For this review, take the finished solid that the model builds, in its own axes (mm). A direction names the side the tool comes from. Coordinates: 2 decimals unless noted, no trailing zeros. Loops run counter-clockwise (first coordinate to the right, second up) from the corner with the lowest first, then second, coordinate; pieces in that order, holes last. Notation, with made-up numbers: (-9, 6.5) -> (39, 6.5) arc R37 ccw to (39, 45.5) -> close; hole circle Ø9 at (7.25, -24). An arc over 180 degrees is marked (long way). Answer in a Markdown table with one row per item.
Autodesk Inventor part; units mm, degrees
ref_plane "YZ Plane" through (0, 0, 0) normal (1, 0, 0) x (0, 1, 0)
ref_plane "XZ Plane" through (0, 0, 0) normal (0, 1, 0) x (-1, 0, 0)
ref_plane "XY Plane" through (0, 0, 0) normal (0, 0, 1) x (1, 0, 0)
sketch "Sketch1" plane through (0, 0, 0) normal (0, 1, 0) x (-1, 0, 0)
  line L0 (0, 0) -> (12.7, 0)
  line L1 (12.7, 0) -> (12.7, 38.1)
  line L2 (12.7, 38.1) -> (0, 38.1)
  line L3 (0, 38.1) -> (0, 0)
  circle A0 centre (6.35, 31.75) radius 2.5797
  circle A1 centre (6.35, 6.35) radius 2.5797
  line L4 (0, 0) -> (127, 0)
  line L5 (127, 0) -> (127, 3.175)
  line L6 (127, 3.175) -> (0, 3.175)
  line L7 (0, 3.175) -> (0, 0)
  line L8 (12.7, 38.1) -> (127, 3.175)
  line L9 (0, 3.175) -> (127, 3.175)
  line L10 (127, 3.175) -> (127, 1.5875)
  line L11 (127, 1.5875) -> (0, 1.5875)
  line L12 (0, 1.5875) -> (0, 3.175)
  line L13 (0, 3.175) -> (19.05, 3.175)
  line L14 (19.05, 3.175) -> (19.05, 1.5875)
  line L15 (19.05, 1.5875) -> (0, 1.5875)
  line L16 (0, 1.5875) -> (0, 3.175)
  line L17 (127, 3.175) -> (120.65, 3.175)
  line L18 (120.65, 3.175) -> (120.65, 1.5875)
  line L19 (120.65, 1.5875) -> (127, 1.5875)
  line L20 (127, 1.5875) -> (127, 3.175)
  line L21 (120.65, 3.175) -> (120.65, 5.1153)
  line L22 (127, 0) -> (0, 0)
  line L23 (0, 0) -> (0, -12.7)
  line L24 (0, -12.7) -> (127, -12.7)
  line L25 (127, -12.7) -> (127, 0)
  line L26 (120.65, 1.5875) -> (120.65, 0)
  line L27 (19.05, 1.5875) -> (19.05, 0)
  point P0 (0, 3.175)
  point P1 (0, 1.5875)
  point P2 (120.65, 1.5875)
  point P3 (120.65, 3.175)
  point P4 (19.05, 3.175)
  point P5 (19.05, 1.5875)
  point P6 (120.65, 3.175)
  point P7 (12.7, 1.5875)
  point P8 (12.7, 3.175)
  dimension "d0" = 12.7
  dimension "d1" = 6.35
  dimension "d2" = 6.35
  dimension "d3" = 25.4
  dimension "d5" = 6.35
  dimension "d6" = 5.1594
  dimension "d7" = 127
  dimension "d8" = 3.175
  dimension "d9" = 127
  dimension "d10" = 1.5875
  dimension "d15" = 19.05
  dimension "d16" = 1.5875
  dimension "d17" = 6.35
  dimension "d18" = 1.5875
  dimension "d25" = 12.7
  dimension "d27" = 6.35
extrude "Extrusion1" add sketch "Sketch1" along normal blind 3.175 contours L3 L11 L1 L0 | L3 L6 L1 L11 | L3 L2 L1 L6 | L1 L8 L21 L6
extrude "Extrusion2" add sketch "Sketch1" along normal up to surface (3.175 mm away) contours L27 L11 L26 L4 | L14 L6 L18 L11
fillet "Fillet1" radius 3.175 3 edges at (-12.7, 1.5875, 0) (0, 1.5875, 0) (0, 1.5875, 38.1)
equation "\"d1\" = d5"
equation "\"d2\" = d21"
equation "\"d5\" = 0.5 * d0"
equation "\"d16\" = d18"
equation "\"d21\" = d5"
properties part number "Gripper triangle"
Item 1: Take a section at A-A, the plane y = 0.6. Count the separate pieces of the cut face and the enclosed holes in it, and give its area (3 significant figures).
Worked answers:
| item | result |
|---|---|
| separate pieces | 1 |
| enclosed holes | 2 |
| area | 2,750 mm² |
Item 2: Take a section at D-D, the plane z = 6.35. State the section outline as (x, y) points (3 decimals).
Worked answers:
| item | result |
|---|---|
| outline | (-116.609, 0) -> (-8.93, 0) -> (-8.93, 3.175) -> (-116.609, 3.175) -> close; (-3.77, 0) -> (0, 0) -> (0, 3.175) -> (-3.77, 3.175) -> close |
Item 3: Insertion check: pin 1 (4.5 mm diameter, centred on x = -6.35, z = 6.35, fed in from +Y); pin 2 (1.6 mm diameter, centred on y = 1, z = 1, fed in from +X). Each pin has a flat end and moves straight along its axis. Give the tip position at first contact, or say it passes through.
Worked answers:
| item | result |
|---|---|
| pin 1 | through |
| pin 2 | x = -0.31 |
Item 4: Take a section at C-C, the plane z = 30.5. State the section outline as (x, y) points (3 decimals).
Worked answers:
| item | result |
|---|---|
| outline | (-37.573, 0) -> (-8.607, 0) -> (-8.607, 3.175) -> (-37.573, 3.175) -> close; (-4.093, 0) -> (0, 0) -> (0, 3.175) -> (-4.093, 3.175) -> close |
Item 5: The part is to be moulded in two halves that separate along Z. For faces 1 (the cylindrical face through (-0.91, 1.61, 0.95)), 2 (the flat face through (-46, 0, 15)), 3 (the cylindrical face through (-0.95, 1.61, 37.19)), 4 (the cylindrical face through (-5.79, 1.57, 34.27)), say which applies: +Z half, -Z half, draft (parallel to the pull), parting line (faces both ways), or undercut.
Worked answers:
| item | result |
|---|---|
| face 1 | -Z half |
| face 2 | draft |
| face 3 | +Z half |
| face 4 | undercut |
Item 6: Take a section at B-B, the plane x = -6.35. State the section outline as (y, z) points (3 decimals).
Worked answers:
| item | result |
|---|---|
| outline | (0, 0) -> (3.175, 0) -> (3.175, 3.77) -> (0, 3.77) -> close; (0, 8.93) -> (3.175, 8.93) -> (3.175, 29.17) -> (0, 29.17) -> close; (0, 34.33) -> (3.175, 34.33) -> (3.175, 38.1) -> (0, 38.1) -> close |
Item 7: For faces 5 (the flat face through (-19.05, 2, 2)), 6 (the flat face through (-8, 2, 38.1)), list the 3-axis set-ups (+Z, -Z, +X, -X, +Y, -Y) from which the entire face can be reached by the end or side of a thin tool; tool diameter is ignored.
Worked answers:
| item | result |
|---|---|
| face 5 | -Z, +Y, -Y |
| face 6 | +Z, +X, -X, +Y, -Y |
Item 8: For L1, parallel to Z at x = -6.35, y = 1.3; L2, parallel to Z at x = -57, y = 2.85; L3, parallel to Z at x = -101, y = 2, list the stretches that pass through material, from the lowest coordinate up.
Worked answers:
| item | result |
|---|---|
| L1 | 0 to 3.77, 8.93 to 29.17, 34.33 to 38.1 |
| L2 | 0 to 24.56 |
| L3 | 0 to 11.12 |
